```python
from build123d import *

# Parameters (mm, degrees)
F0_R     = 1.6
F0_W     = 12.72
F0_H     = 12.72
F1_DEPTH = 6
F2_R     = 35
F3_R     = 20


with BuildPart() as f1:
    # F0 (on Top) → F1 (new body)
    with BuildSketch(Plane.XY):
        Polygon((27.6, 119.208467), (-14.4, 69.6), (-14.4, -14.4), (69.6, -14.4), (69.6, 69.6), align=None)
        with Locations((27.6, -7.2)):
            Circle(F0_R, mode=Mode.SUBTRACT)
        Polygon((27.6, 0), (16.167706, 0), (8.083853, 8.083853), (0, 16.167706), (0, 27.6), (0, 39.032294), (8.083853, 47.116147), (16.167706, 55.2), (27.6, 55.2), (39.032294, 55.2), (47.116147, 47.116147), (55.2, 39.032294), (55.2, 27.6), (55.2, 16.167706), (47.116147, 8.083853), (39.032294, 0), align=None, mode=Mode.SUBTRACT)
        with Locations((9.6, 69.6)):
            Circle(F0_R, mode=Mode.SUBTRACT)
        with Locations((45.6, 69.6)):
            Circle(F0_R, mode=Mode.SUBTRACT)
        with Locations((27.6, 91.96)):
            Rectangle(F0_W, F0_H, mode=Mode.SUBTRACT)
    extrude(amount=F1_DEPTH)

    # F2
    f2_edges = [f1.edges().sort_by_distance(p)[0] for p in [
        (69.6, -14.4, 3),
        (-14.4, -14.4, 3),
        (-14.4, 69.6, 3),
        (69.6, 69.6, 3),
    ]]
    fillet(f2_edges, radius=F2_R)

    # F3
    f3_edges = [f1.edges().sort_by_distance(p)[0] for p in [
        (27.6, 119.208467, 3),
    ]]
    fillet(f3_edges, radius=F3_R)


solid = f1.part
```
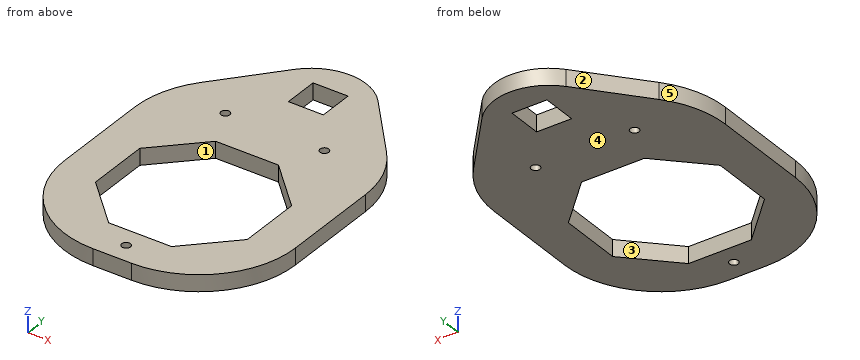
Input: part model. Units: mm. Frame: model coordinates. Face numbers are marked on the shaded views. A direction names the side the tool comes from. Round coordinates to 2 decimals unless told otherwise and drop trailing zeros. Write each loop counter-clockwise with the first axis right and the second up, starting at its lowest first coordinate (ties: lowest second). Pieces come first, ordered by that corner, then holes. Notation, with made-up numbers: M -39.75,59 L -5.75,59 A31 ccw -5.75,98 Z; hole C -4,57 d6. An arc over 180 degrees is marked long. Write each question's results on one line, items separated by ' | '.
Q1. Section query B-B (y = 6). Return loops of the section in (x, z), and give its area (3 significant figures).
Results:
outline: M -11.21,0 L 10.17,0 L 10.17,6 L -11.21,6 Z; M 45.03,0 L 66.41,0 L 66.41,6 L 45.03,6 Z | area: 257 mm^2
Q2. Draft query along Y for the marked faces 3, 4 and 5. Return one class per face: released by +Y, released by -Y, zero draft, split by the parting line, or undercut.
Results:
face 3: undercut | face 4: zero draft | face 5: released by +Y
Q3. Section query C-C (x = 9.6). Return loops of the section in (y, z), and give its area (3 significant figures).
Results:
outline: M -12.63,0 L 6.57,0 L 6.57,6 L -12.63,6 Z; M 48.63,0 L 68,0 L 68,6 L 48.63,6 Z; M 71.2,0 L 97.95,0 L 97.95,6 L 71.2,6 Z | area: 392 mm^2
Q4. Access query for the marked faces 1 and 2. Directions: +Z, -Z, +X, -X, +Y, -Y. A direction counts if a zero-diameter tool reaches every point of the face in a straight line with its end or side. Return the directions, or none.
Results:
face 1: +Z, -Z | face 2: +Z, -Z, -X, +Y
Q5. Pin query (flat end, axial travel): P1, Ø1.8, axis at y = 91, z = 3, coming from the +X side; P2, Ø1.8, axis at x = 26.5, z = 2, coming from the +Y side; P3, Ø1.8, axis at y = 95, z = 3, coming from the -X side. Return the tip coordinate at first contact, or that it passes through.
Results:
P1: stops at x = 52.24 | P2: stops at y = 108.26 | P3: stops at x = 6.34
Q6. Section query D-D (y = 69.6). Return loops of the section in (x, z), and give its area (3 significant figures).
Results:
outline: M -11.97,0 L 8,0 L 8,6 L -11.97,6 Z; M 11.2,0 L 44,0 L 44,6 L 11.2,6 Z; M 47.2,0 L 67.17,0 L 67.17,6 L 47.2,6 Z | area: 436 mm^2
Q7. Line query: line 1 along Y through (x, z) = (27.6, 4.45); line 2 along X through (y, z) = (36, 1.6); line 3 along Y through (x, z) = (45, 1.8). Output: solid intervals per line, ascending.
Results:
line 1: y = -14.4 to -8.8, -5.6 to 0, 55.2 to 85.6, 98.32 to 108.26 | line 2: x = -14.4 to 0, 55.2 to 69.6 | line 3: y = -12.82 to 5.97, 49.23 to 68.12, 71.08 to 98.66
Q8. Section query A-A (z = 3.1). Return loops of the section in (x, y).
Results:
outline: M -14.4,20.6 A35 ccw 20.6,-14.4 L 34.6,-14.4 A35 ccw 69.6,20.6 L 69.6,56.77 A35 ccw 61.31,79.39 L 42.86,101.18 A20 ccw 12.34,101.18 L -6.11,79.39 A35 ccw -14.4,56.77 Z; hole M 0,16.17 L 16.17,0 L 39.03,0 L 55.2,16.17 L 55.2,39.03 L 39.03,55.2 L 16.17,55.2 L 0,39.03 Z; hole C 9.6,69.6 d3.2; hole M 21.24,85.6 L 33.96,85.6 L 33.96,98.32 L 21.24,98.32 Z; hole C 27.6,-7.2 d3.2; hole C 45.6,69.6 d3.2
